Design review of the part built by this model. Coordinates are the model's own, in mm. A direction names the side the tool comes from. Coordinates: 2 decimals unless noted, no trailing zeros. Loops run counter-clockwise (first coordinate to the right, second up) from the corner with the lowest first, then second, coordinate; pieces in that order, holes last. Notation, with made-up numbers: M 5.25,48 L 54.25,48 A11 ccw 54.25,63 Z; hole C 15,11.25 d9. An arc over 180 degrees is marked long. Answer as a JSON object with one key per item and string values. Group by question number.
1. Draft analysis for pull direction X (two halves, no side actions). For faces 6 (the flat face through (-87.6, 0, 0)), 7 (the flat face through (1.2, 2, -9)), 8 (the cylindrical face through (1.859, 2.703, 8.584)), 9 (the cylindrical face through (-0.4, -9.76, -2.17)), state which applies: +X half, -X half, draft (parallel to the pull), parting line (faces both ways), or undercut.
2. To check wall thickness, follow probe 1 along X at (y, z) = (-30.5, 37.5); probe 2 along Z at (x, y) = (-33.5, -1.5). State the ranges of each line that lie inside material, in increasing order.
3. Insertion check: pin 1 (10 mm diameter, centred on x = -57, z = 3, fed in from -Y); pin 2 (5 mm diameter, centred on y = -16, z = -33, fed in from -X); pin 3 (12 mm diameter, centred on x = -34.5, z = 11.5, fed in from -Y). Each pin has a flat end and moves straight along its axis. Give the tip position at first contact, or say it passes through.
4. Consider section C-C (x = -50). State the section outline as (y, z) points.
5. Machinability: for faces 1 (the flat face through (2.5, 2, 9)), 2 (the flat face through (7.2, 1, -1)), 3 (the flat face through (6.2, 13, -56)), 4 (the cylindrical face through (5.58, -35.14, -45.83)), 5 (the flat face through (4.7, -38, -42)), which of the approach directions +Z, -Z, +X, -X, +Y, -Y give a long, thin tool a straight path to every point of the face, cutting with its end or side? Answer none if there is none.
from build123d import *

# Parameters (mm, degrees)
SKETCH4_R           = 8.5
BOSS_EXTRUDE2_DEPTH = 84.8
CHAMFER2_SIZE       = 0.272977676
CHAMFER2_SIZE2      = 0.75
FILLET1_R           = 0.25


with BuildPart() as part:
    # Sketch1 → Revolve1 (revolve)
    with BuildSketch(Plane(origin=(0, 0, 0), x_dir=(-1, 0, 0), z_dir=(0, 0, -1)), mode=Mode.PRIVATE) as revolve1_sk:
        Polygon((-7.2, 56.065405665), (-7.2, 0), (2.8, 0), (2.8, 10), (-1.2, 10), (-1.2, 9), (-2.5, 9), (-2.5, 10), (-3.7, 10), (-3.7, 56.25), (-4.7, 56.25), (-4.7, 57.75), (-6.2, 57.75), (-6.2, 57.1), align=None)
    revolve(revolve1_sk.sketch.rotate(Axis((7.200025, 0, 0), (-1, 0, 0)), 270), axis=Axis((7.200025, 0, 0), (-1, 0, 0)))

    # Sketch4 → Boss-Extrude2 (add)
    with BuildSketch(Plane.ZY.offset(2.8)):
        Circle(SKETCH4_R)
    extrude(amount=BOSS_EXTRUDE2_DEPTH)

    # Chamfer2
    chamfer2_edges = [part.edges().sort_by_distance(p)[0] for p in [
        (-2.8, 0, -10),
    ]]
    chamfer2_side = [part.faces().sort_by_distance(p)[0] for p in [
        (-2.8, 0, -9.717157288),
    ]]
    chamfer(chamfer2_edges, length=CHAMFER2_SIZE, length2=CHAMFER2_SIZE2, reference=chamfer2_side[0])

    # Fillet1
    fillet1_edges = [part.edges().sort_by_distance(p)[0] for p in [
        (4.7, 0, -57.75),
    ]]
    fillet(fillet1_edges, radius=FILLET1_R)


solid = part.part
Findings below:
{
 "1": {"face 6": "-X half", "face 7": "undercut", "face 8": "undercut", "face 9": "draft"},
 "2": {"probe 1": "x = 3.7 to 7.2", "probe 2": "z = -8.37 to 8.37"},
 "3": {"pin 1": "stops at y = -8.5", "pin 2": "stops at x = 3.7", "pin 3": "stops at y = -6.48"},
 "4": {"outline": "C 0,0 d17"},
 "5": {"face 1": "none", "face 2": "+Z, -Z, +X, +Y, -Y", "face 3": "+X", "face 4": "+X, -X", "face 5": "-X"}
}
